Answer from the drawing. Dimensions are ordinates in mm from the lowest x, y and z of the part. A direction names the side the tool comes from. Round coordinates to 2 decimals unless told otherwise and drop trailing zeros. Write each loop counter-clockwise with the first axis right and the second up, starting at its lowest first coordinate (ties: lowest second). Pieces come first, ordered by that corner, then holes. Notation, with made-up numbers: (-2.75, 73) - (30.25, 73) arc R14 ccw to (30.25, 81) - close; hole circle Ø2 at (-32, 39). An arc over 180 degrees is marked (long way). Use a Markdown table: item, result. Add a question column.
1) A cutting plane is placed at C-C (x = 45.5). Give the vertices of the cut face in (y, z).
2) A cutting plane is placed at A-A (z = 10). Give the vertices of the cut face in (x, y).
3) A cutting plane is placed at D-D (y = 16). Give the vertices of the cut face in (x, z), then the cut area to 3 significant figures.
4) A tool of negligible diameter and unlimited length cuts with its end or side. For the marked faces 1, 2 and 3, from which of +Z, -Z, +X, -X, +Y, -Y can it reach the whole face along a straight path? Write none if from no direction.
5) Find the intervals of material crossed by probe 1 along X at (y, z) = (3, 16.5); probe 2 along Y at (x, z) = (24, 13.25); probe 3 along Z at (x, y) = (18, 12.25), in increasing order. Write a range as from..to.
6) Each of these flat-tipped pins is pushed along its axis until it touches: P1, Ø12, axis at x = 9, y = 17.5, coming from the +Z side; P2, Ø1, axis at x = 24.5, z = 12, coming from the +Y side; P3, Ø5, axis at x = 43, z = 13, coming from the +Y side. Where does it stop, or does it pass through?
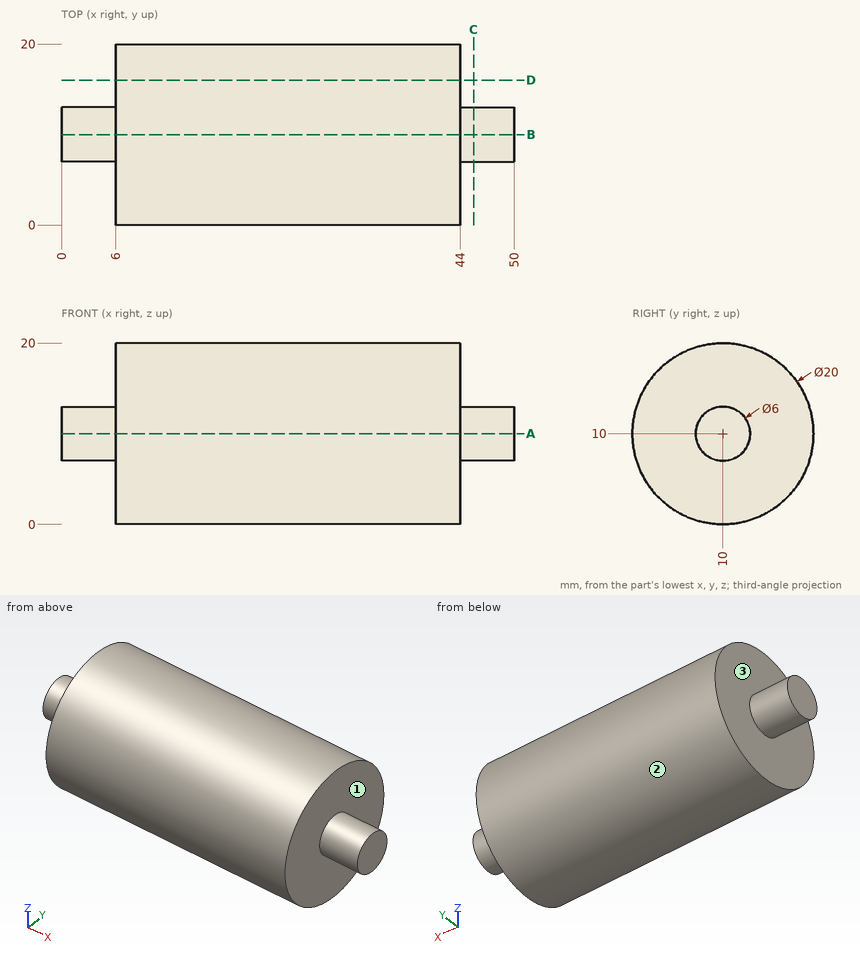
Entries:
| question | item | result |
|---|---|---|
| 1 | outline | circle Ø6 at (10, 10) |
| 2 | outline | (0, 7) - (6, 7) - (6, 0) - (44, 0) - (44, 7) - (50, 7) - (50, 13) - (44, 13) - (44, 20) - (6, 20) - (6, 13) - (0, 13) - close |
| 3 | outline | (6, 2) - (44, 2) - (44, 18) - (6, 18) - close |
| 3 | area | 608 mm² |
| 4 | face 1 | +X |
| 4 | face 2 | +X, -X |
| 4 | face 3 | -X |
| 5 | probe 1 | x = 6..44 |
| 5 | probe 2 | y = 0.54..19.46 |
| 5 | probe 3 | z = 0.26..19.74 |
| 6 | P1 | stops at z = 19.89 |
| 6 | P2 | stops at y = 19.89 |
| 6 | P3 | stops at y = 19.99 |
